from build123d import *

# Parameters (mm, degrees)
CHANFREIN1_SIZE = 0.5
CHANFREIN2_SIZE = 0.5


with BuildPart() as part:
    # Esquisse1 → Révolution1 (revolve)
    with BuildSketch(Plane(origin=(0, 0, 0), x_dir=(0, 0, -1), z_dir=(1, 0, 0)), mode=Mode.PRIVATE) as r_volution1_sk:
        Polygon((0, 10.5), (0, 5.13), (5.06, 5.13), (5.06, 7), (2.4, 7), (2.4, 10.5), align=None)
    revolve(r_volution1_sk.sketch.rotate(Axis((0, 0, 0), (0, 0, -1)), 90), axis=Axis((0, 0, 0), (0, 0, -1)))  # turned: the seam where the file's is

    # Chanfrein1
    chanfrein1_edges = [part.edges().sort_by_distance(p)[0] for p in [
        (-5.13, 0, 0),
    ]]
    chamfer(chanfrein1_edges, length=CHANFREIN1_SIZE)

    # Chanfrein2
    chanfrein2_edges = [part.edges().sort_by_distance(p)[0] for p in [
        (-5.13, 0, -5.06),
    ]]
    chamfer(chanfrein2_edges, length=CHANFREIN2_SIZE)


solid = part.part
Input: part model. Units: mm. Frame: model coordinates. Give positions to 0.01 mm unless a question says otherwise; leave off trailing zeros. Write each loop counter-clockwise with the first axis right and the second up, starting at its lowest first coordinate (ties: lowest second). Pieces come first, ordered by that corner, then holes. Notation, with made-up numbers: M 43.5,39 L 99.5,39 A19 cw 99.5,67 Z; hole C -19,-31 d7. An arc over 180 degrees is marked long. Write item = value, one per line. Start each with the question number.
1) Cut plane C-C on z = -1.25. Return the cut outline in (x, y), then the cut area to 3 significant figures.
2) Cut plane A-A on y = 0. Return the cut outline in (x, z), then the cut area to 3 significant figures.
3) Draft query along Y for faces 1 (the cylindrical face through (3.23, 6.21, -3.71)), 2 (the cylindrical face through (-4.07, 3.12, -2.56)), 3 (the flat face through (-2, 7, -2.4)). Return one class per face: +Y half, -Y half, draft (parallel to the pull), parting line (faces both ways), or undercut.
4) Material intervals for line 1 along Y through (x, z) = (0, -3.25); line 2 along Y through (x, z) = (0, -2.1); line 3 along Z through (x, y) = (-1, -7.25), sorted ascending. Write a range as [from, to].
5) First-contact query: pin 1 Ø1 at (y, z) = (5.5, -2.5) entering from -X; pin 2 Ø1 at (y, z) = (-1.5, -3.5) entering from -X; pin 3 Ø1 at (x, z) = (-4, -2) entering from +Y. Flat tips, straight axial feed; report the tip coordinate or a pass-through.
6) Cut plane D-D on y = -6. Return the cut outline in (x, z).
Solved:
q1.outline = C 0,0 d21; hole C 0,0 d10.26
q1.area = 264 mm2
q2.outline = M -10.5,-2.4 L -7,-2.4 L -7,-5.06 L -5.63,-5.06 L -5.13,-4.56 L -5.13,-0.5 L -5.63,0 L -10.5,0 Z; M 5.13,-4.56 L 5.63,-5.06 L 7,-5.06 L 7,-2.4 L 10.5,-2.4 L 10.5,0 L 5.63,0 L 5.13,-0.5 Z
q2.area = 35.2 mm2
q3.face_1 = parting line
q3.face_2 = undercut
q3.face_3 = draft
q4.line_1 = [-7, -5.13], [5.13, 7]
q4.line_2 = [-10.5, -5.13], [5.13, 10.5]
q4.line_3 = [-2.4, 0]
q5.pin_1 = -9.23
q5.pin_2 = -6.93
q5.pin_3 = 9.9
q6.outline = M -8.62,-2.4 L -3.61,-2.4 L -3.61,-5.06 L 3.61,-5.06 L 3.61,-2.4 L 8.62,-2.4 L 8.62,0 L -8.62,0 Z
